```python
from build123d import *

# Parameters (mm, degrees)
F0_R            = 45
F0_R_2          = 22.5
F1_DEPTH        = 100
F2_SIZE         = 20
F3_SIZE         = 3
F4_W            = 48.8546937704
F4_H            = 132.6055675745
F5_DEPTH        = 100
F8_D            = 4
F8_DEPTH        = 25
F8_TIP          = 1.2017212381
F10_D           = 6
F10_CBORE_D     = 11.25
F10_CBORE_DEPTH = 35


with BuildPart() as f1:
    # F0 (on Top) → F1 (new body)
    with BuildSketch(Plane.XY):
        Circle(F0_R)
        Circle(F0_R_2, mode=Mode.SUBTRACT)
    extrude(amount=F1_DEPTH)

    # F2
    f2_edges = [f1.edges().sort_by_distance(p)[0] for p in [
        (-45, 0, 100),
    ]]
    chamfer(f2_edges, length=F2_SIZE)

    # F3
    f3_edges = [f1.edges().sort_by_distance(p)[0] for p in [
        (-45, 0, 0),
        (-22.5, 0, 0),
    ]]
    chamfer(f3_edges, length=F3_SIZE)

    # F4 (on Top) → F5 (cut)
    with BuildSketch(Plane.XY):
        with Locations((24.4273468852, 2.2433325648)):
            Rectangle(F4_W, F4_H)
    extrude(amount=F5_DEPTH, mode=Mode.SUBTRACT)

    # F8
    with Locations(Plane.YZ):
        with Locations((34, 68), (34, 16)):
            Hole(F8_D / 2, depth=F8_DEPTH)
            with Locations((0, 0, -(F8_DEPTH + F8_TIP / 2))):  # 118° drill point
                Cone(0, F8_D / 2, F8_TIP, mode=Mode.SUBTRACT)

    # F10 (through all)
    with Locations(Plane(origin=(-50, 0, 0), x_dir=(0, 1, 0), z_dir=(-1, 0, 0))):
        with Locations((-34, -68), (-34, -16)):
            CounterBoreHole(F10_D / 2, F10_CBORE_D / 2, F10_CBORE_DEPTH)


solid = f1.part
```
Check sheet for the modelled part. Datum: model origin and axes. Units: mm. A direction names the side the tool comes from. Round coordinates to 2 decimals unless told otherwise and drop trailing zeros. Loops run counter-clockwise (first coordinate to the right, second up) from the corner with the lowest first, then second, coordinate; pieces in that order, holes last. Notation, with made-up numbers: (75.5, 67) -> (99.5, 67) arc R20 ccw to (99.5, 98) -> close; hole circle Ø2 at (-22.75, 7.5). An arc over 180 degrees is marked (long way). Write item = value, one per line. Start each with the question number.
1) Sectioned sample at C-C, the plane z = 81.5. Record the cut outline in (x, y), plus the area to 3 significant figures.
2) Release check for a two-part mould opening along Y. For faces 1 (the flat face through (0, 34, 49)), 2 (the cylindrical face through (-22.89, -28.8, 18.15)), 3 (the cylindrical face through (-44.99, 0.99, 40.96)) record: released by +Y, released by -Y, zero draft, split by the parting line, or undercut.
3) Set-up check for faces 4 (the flat face through (-15, -31.6, 18.4)), 5 (the cylindrical face through (-12.675, 32.925, 17.686)), 6 (the conical face through (-28.187, 0.62, 96.807)): record each of +Z, -Z, +X, -X, +Y, -Y from which the full face is reachable in a straight line by a thin tool's end or side.
4) Thickness scan on probe 1 along Z at (x, y) = (-12, 34); probe 2 along Z at (x, y) = (-22.75, -34) (3 decimals); probe 3 along Y at (x, z) = (-12.25, 16). Record the ranges inside material, lowest first.
5) Gauge pin test, flat ends, axial feed: pin 1 Ø6.5 at (y, z) = (34, 68) entering from -X; pin 2 Ø1.5 at (x, z) = (-32.5, 67.5) entering from -Y; pin 3 Ø3 at (x, z) = (-19, 39.5) entering from +Y. Record the tip position at first contact, or that the pin passes through.
6) Sectioned sample at B-B, the plane y = 0. Record the cut outline in (x, z).
7) Sectioned sample at A-A, the plane x = -11. State how many separate pieces and enclosed holes the cut face has, plus the area to 3 significant figures.
Results are:
q1.outline = (0, -43.5) -> (0, -22.5) arc R22.5 cw to (0, 22.5) -> (0, 43.5) arc R43.5 ccw to start
q1.area = 2,180 mm^2
q2.face_1 = zero draft
q2.face_2 = undercut
q2.face_3 = split by the parting line
q3.face_4 = -X
q3.face_5 = +X
q3.face_6 = +Z, -X
q4.probe_1 = 0 to 14, 18 to 66, 70 to 88.94
q4.probe_2 = 0 to 10.375, 21.625 to 62.375, 73.625 to 84.091
q4.probe_3 = -43.3 to -37, -31 to -18.87, 18.87 to 32, 36 to 43.3
q5.pin_1 = -32.85
q5.pin_2 = -28.52
q5.pin_3 = 41.46
q6.outline = (-45, 3) -> (-42, 0) -> (-25.5, 0) -> (-22.5, 3) -> (-22.5, 100) -> (-25, 100) -> (-45, 80) -> close
q7.separate_pieces = 2
q7.enclosed_holes = 4
q7.area = 4,280 mm^2
